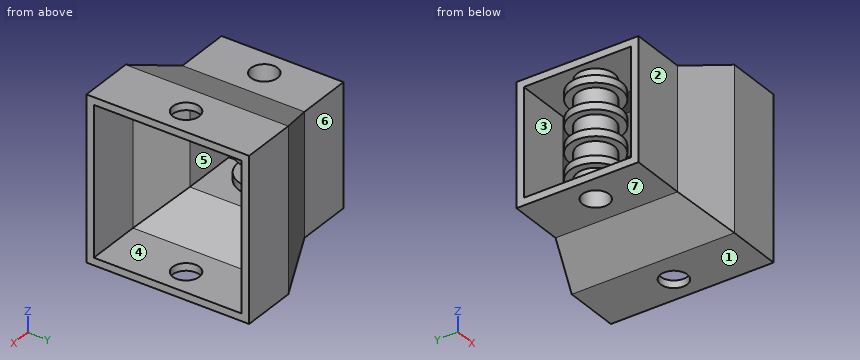
from build123d import *

# Parameters (mm, degrees)
SKETCH_1_R               = 2.5
EXTRUDE_1_DEPTH          = 1.5
SKETCH_2_R               = 3.5
EXTRUDE_2_DEPTH          = 1
SKETCH_3_R               = 2.5
EXTRUDE_3_DEPTH          = 2.5
SKETCH_4_R               = 3.5
EXTRUDE_4_DEPTH          = 1
SKETCH_5_R               = 2.5
EXTRUDE_5_DEPTH          = 2.5
SKETCH_6_R               = 3.5
EXTRUDE_6_DEPTH          = 1
SKETCH_7_R               = 2.5
EXTRUDE_7_DEPTH          = 2.5
SKETCH_10_R              = 3.5
EXTRUDE_9_DEPTH          = 1
SKETCH_11_R              = 2.5
EXTRUDE_10_DEPTH         = 1.5
SKETCH_12_R              = 1.8
CUT_EXTRUDE_2_DEPTH      = 15.5
SKETCH_13_W              = 22
SKETCH_13_H              = 22
SKETCH_13_W_2            = 20
SKETCH_13_H_2            = 20
EXTRUDE_11_DEPTH         = 3.5
EXTRUDE_11_DEPTH_BACK    = 4
SKETCH_14_W              = 16.5
SKETCH_14_H              = 16.5
SKETCH_14_W_2            = 14.5
SKETCH_14_H_2            = 14.5
EXTRUDE_12_DEPTH         = 4
EXTRUDE_12_DEPTH_BACK    = 3.5
PATTERN_CIRCULAR_1_COUNT = 4
SKETCH_19_R              = 1.8
CUT_EXTRUDE_3_DEPTH      = 20.2500001
SKETCH_20_R              = 1.8
CUT_EXTRUDE_4_DEPTH      = 23.0000001


with BuildPart() as part:
    # Sketch 1 → Extrude 1 (new body)
    with BuildSketch(Plane.XY):
        Circle(SKETCH_1_R)
    extrude(amount=EXTRUDE_1_DEPTH)

    # Sketch 2 → Extrude 2 (add)
    with BuildSketch(Plane.XY.offset(1.5)):
        Circle(SKETCH_2_R)
    extrude(amount=EXTRUDE_2_DEPTH)

    # Sketch 3 → Extrude 3 (add)
    with BuildSketch(Plane.XY.offset(2.5)):
        Circle(SKETCH_3_R)
    extrude(amount=EXTRUDE_3_DEPTH)

    # Sketch 4 → Extrude 4 (add)
    with BuildSketch(Plane.XY.offset(5)):
        Circle(SKETCH_4_R)
    extrude(amount=EXTRUDE_4_DEPTH)

    # Sketch 5 → Extrude 5 (add)
    with BuildSketch(Plane.XY.offset(6)):
        Circle(SKETCH_5_R)
    extrude(amount=EXTRUDE_5_DEPTH)

    # Sketch 6 → Extrude 6 (add)
    with BuildSketch(Plane.XY.offset(8.5)):
        Circle(SKETCH_6_R)
    extrude(amount=EXTRUDE_6_DEPTH)

    # Sketch 7 → Extrude 7 (add)
    with BuildSketch(Plane.XY.offset(9.5)):
        Circle(SKETCH_7_R)
    extrude(amount=EXTRUDE_7_DEPTH)

    # Sketch 10 → Extrude 9 (add)
    with BuildSketch(Plane.XY.offset(12)):
        Circle(SKETCH_10_R)
    extrude(amount=EXTRUDE_9_DEPTH)

    # Sketch 11 → Extrude 10 (add)
    with BuildSketch(Plane.XY.offset(13)):
        Circle(SKETCH_11_R)
    extrude(amount=EXTRUDE_10_DEPTH)

    # Sketch 12 → Cut-Extrude 2 (cut, through all)
    with BuildSketch(Plane.XY.offset(14.5)):
        Circle(SKETCH_12_R)
    extrude(amount=-CUT_EXTRUDE_2_DEPTH, mode=Mode.SUBTRACT)

    # Sketch 14 → Extrude 12 (add, two sides)
    with BuildSketch(Plane(origin=(0, 0, 0), x_dir=(0, 0, -1), z_dir=(1, 0, 0))) as extrude_12_sk:
        with Locations((-7.25, 0)):
            Rectangle(SKETCH_14_W, SKETCH_14_H)
        with Locations((-7.25, 0)):
            Rectangle(SKETCH_14_W_2, SKETCH_14_H_2, mode=Mode.SUBTRACT)
    extrude(amount=EXTRUDE_12_DEPTH)
    extrude(extrude_12_sk.sketch, amount=-EXTRUDE_12_DEPTH_BACK)



with BuildPart() as body_2:
    # Sketch 13 → Extrude 11 (new body, two sides)
    with BuildSketch(Plane(origin=(15, 0, 0), x_dir=(0, 0, -1), z_dir=(1, 0, 0))) as extrude_11_sk:
        with Locations((-7.25, 0)):
            Rectangle(SKETCH_13_W, SKETCH_13_H)
        with Locations((-7.25, 0)):
            Rectangle(SKETCH_13_W_2, SKETCH_13_H_2, mode=Mode.SUBTRACT)
    extrude(amount=EXTRUDE_11_DEPTH)
    extrude(extrude_11_sk.sketch, amount=-EXTRUDE_11_DEPTH_BACK)


with BuildPart() as part_1:
    add(part.part)

    add(body_2.part)  # Loft 2 merges body 2
    # Sketch 16 → Loft 2 section 0
    with BuildSketch(Plane.ZY.offset(-11)):
        Polygon((-3.75, 11), (-2.75, 10), (17.25, 10), (18.25, 11), align=None)
    # Sketch 17 → Loft 2 section 1
    with BuildSketch(Plane(origin=(4, 0, 0), x_dir=(0, 0, -1), z_dir=(1, 0, 0))):
        Polygon((-15.5, 8.25), (-14.5, 7.25), (0, 7.25), (1, 8.25), align=None)
    loft_2 = loft()

    # Pattern Circular 1: Loft 2 ×4 about axis
    pattern_circular_1_axis = Axis((0, 0, 7.25), (1, 0, 0))
    for i in range(1, PATTERN_CIRCULAR_1_COUNT):
        add(loft_2.rotate(pattern_circular_1_axis, i * 360 / PATTERN_CIRCULAR_1_COUNT))

    # Sketch 19 → Cut-Extrude 3 (cut, through all)
    with BuildSketch(Plane.XY.offset(15.5)):
        Circle(SKETCH_19_R)
    extrude(amount=-CUT_EXTRUDE_3_DEPTH, mode=Mode.SUBTRACT)

    # Sketch 20 → Cut-Extrude 4 (cut, through all)
    with BuildSketch(Plane.XY.offset(18.25)):
        with Locations((15, 0)):
            Circle(SKETCH_20_R)
    extrude(amount=-CUT_EXTRUDE_4_DEPTH, mode=Mode.SUBTRACT)


solid = part_1.part
Input: part model. Units: mm. Frame: model coordinates. Face numbers are marked on the shaded views. A direction names the side the tool comes from. Give positions to 0.01 mm unless a question says otherwise; leave off trailing zeros. Order: outer loops, then holes, each group sorted by start corner. A loop starts at its lowest first (then second) coordinate and runs counter-clockwise, first axis right, second up. Notation, with made-up numbers: (8.25, 51) -> (66.25, 51) arc R27 ccw to (66.25, 87) -> close; hole circle Ø1 at (28.25, 13.5). An arc over 180 degrees is marked (long way). Use one line per item in the form item = value.
1) Section A-A, the plane x = 15. Return loops of the section in (y, z).
Response values:
outline = (-11, -3.75) -> (-1.8, -3.75) -> (-1.8, -2.75) -> (-10, -2.75) -> (-10, 17.25) -> (-1.8, 17.25) -> (-1.8, 18.25) -> (-11, 18.25) -> close; (1.8, -3.75) -> (11, -3.75) -> (11, 18.25) -> (1.8, 18.25) -> (1.8, 17.25) -> (10, 17.25) -> (10, -2.75) -> (1.8, -2.75) -> close
2) Line query: probe 1 along Y at (x, z) = (0, 5.5); probe 2 along Y at (x, z) = (0, 10.25); probe 3 along Y at (x, z) = (15, 17.7). Output: solid intervals per line, ascending.
Response values:
probe_1 = -8.25 to -7.25, -3.5 to -1.8, 1.8 to 3.5, 7.25 to 8.25
probe_2 = -8.25 to -7.25, -2.5 to -1.8, 1.8 to 2.5, 7.25 to 8.25
probe_3 = -11 to -1.8, 1.8 to 11
3) Reachability of the marked faces 4, 5, 6 and 7 from +Z, -Z, +X, -X, +Y, -Y: full face, straight path, thin tool, end or side. Return the list, or none.
Response values:
face_4 = +X
face_5 = +X, -X
face_6 = +Z, -Z, -X, +Y
face_7 = -Z, -X, +Y, -Y
4) First-contact query: pin 1 Ø5 at (y, z) = (2, 6) entering from -X; pin 2 Ø7.5 at (x, y) = (-1.5, 1) entering from +Z; pin 3 Ø6 at (x, y) = (-0.5, 3) entering from -Z; pin 4 Ø10 at (x, z) = (1, 3) entering from -Y. Flat tips, straight axial feed; report the tip coordinate or a pass-through.
Response values:
pin_1 = -3.5
pin_2 = 15.5
pin_3 = -1
pin_4 = -9.04
5) Mould query, pull axis Z, two halves, no side actions, for the marked faces 1, 2 and 3. Classes: pulls with the +Z half, pulls with the -Z half, needs draft (parallel to the pull), parting line crosses it, or undercut.
Response values:
face_1 = pulls with the -Z half
face_2 = needs draft
face_3 = undercut
6) Section B-B, the plane z = 4.5. Count the separate pieces of the cut face and the enclosed holes in it, and give its area (3 significant figures).
Response values:
separate_pieces = 3
enclosed_holes = 1
area = 53.5 mm^2
